Read the model definition and answer for the solid it produces. Units are mm, in the model's axes. Face numbers are marked on the shaded views. Coordinates: 2 decimals unless noted, no trailing zeros. Write each loop counter-clockwise with the first axis right and the second up, starting at its lowest first coordinate (ties: lowest second). Pieces come first, ordered by that corner, then holes.
(1) The part is cut by section C-C, the plane z = 3.5. Determine the outline of the cut face in (x, y), and give its area (3 significant figures).
(2) Given pin 1 (1.5 mm diameter, centred on y = 2, z = -3, fed in from -X), flat-ended and moving along its own axis, determine where the tip first touches the part or whether it passes through.
(3) Straight lines are drawn through the part: line 1 along X through (y, z) = (5.5, 3.5); line 2 along Z through (x, y) = (6, 4.5); line 3 along X through (y, z) = (3, -1.75). For each, find the intervals that lie inside material, in ascending order.
(4) Determine the mould class of the marked faces 1, 2 and 3 for opening direction X: pulls with the +X half, pulls with the -X half, needs draft (parallel to the pull), parting line crosses it, or undercut.
(5) The part is cut by section A-A, the plane y = 3.5. Determine the outline of the cut face in (x, z), and give its area (3 significant figures).
(6) The part is cut by section D-D, the plane x = -10.75. Determine the outline of the cut face in (y, z).
(7) The part is cut by section B-B, the plane x = 5. Determine the outline of the cut face in (y, z), and give its area (3 significant figures).
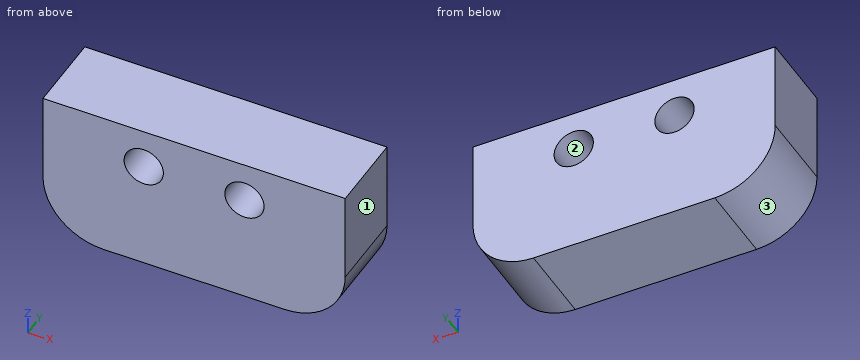
```python
from build123d import *

# Parameters (mm, degrees)
SKETCH_1_W          = 30
SKETCH_1_H          = 15
EXTRUDE_1_DEPTH     = 8
FILLET_1_R          = 6
SKETCH_2_R          = 1.95
CUT_EXTRUDE_1_DEPTH = 19.580904176


with BuildPart() as part:
    # Эскиз1 → Бобышка-Вытянуть1 (new body)
    with BuildSketch(Plane(origin=(0, 0, 0), x_dir=(1, 0, 0), z_dir=(0, 1, 0))):
        Rectangle(SKETCH_1_W, SKETCH_1_H)
    extrude(amount=EXTRUDE_1_DEPTH)

    # Скругление1
    fillet_1_edges = [part.edges().sort_by_distance(p)[0] for p in [
        (-15, 4, -7.5),
        (15, 4, -7.5),
    ]]
    fillet(fillet_1_edges, radius=FILLET_1_R)

    # Эскиз2 → Вырез-Вытянуть1 (cut, through all)
    with BuildSketch(Plane(origin=(0, 8, 0), x_dir=(1, 0, 0), z_dir=(0, 1, 0))):
        with Locations(Location((-5, -3.5, 0), (0, 0, 270))):
            Circle(SKETCH_2_R)
        with Locations(Location((5, -3.5, 0), (0, 0, 270))):
            Circle(SKETCH_2_R)
    extrude(amount=-CUT_EXTRUDE_1_DEPTH, mode=Mode.SUBTRACT)


solid = part.part
```
Computed:
1. outline: (-15, 0) - (-6.95, 0) - (-6.95, 8) - (-15, 8) - close; (-3.05, 0) - (3.05, 0) - (3.05, 8) - (-3.05, 8) - close; (6.95, 0) - (15, 0) - (15, 8) - (6.95, 8) - close
1. area: 178 mm2
2. pin 1: stops at x = -14.95
3. line 1: x = -15 to -6.95, -3.05 to 3.05, 6.95 to 15
3. line 2: z = -7.5 to 1.83, 5.17 to 7.5
3. line 3: x = -14.99 to 14.99
4. face 1: pulls with the +X half
4. face 2: undercut
4. face 3: pulls with the -X half
5. outline: (-15, -1.5) arc R6 ccw to (-9, -7.5) - (9, -7.5) arc R6 ccw to (15, -1.5) - (15, 7.5) - (-15, 7.5) - close; hole circle Ø3.9 at (-5, 3.5); hole circle Ø3.9 at (5, 3.5)
5. area: 411 mm2
6. outline: (0, -7.24) - (8, -7.24) - (8, 7.5) - (0, 7.5) - close
7. outline: (0, -7.5) - (8, -7.5) - (8, 1.55) - (0, 1.55) - close; (0, 5.45) - (8, 5.45) - (8, 7.5) - (0, 7.5) - close
7. area: 88.8 mm2
